Could you check a few things on this model? Use its own coordinates, in mm. A direction names the side the tool comes from. Give positions to 0.01 mm unless a question says otherwise; leave off trailing zeros. Answer in a Markdown table with one row per item. Add a question column.
1. I'm going to push flat-ended pins straight in: pin 1 Ø10.5 at (x, y) = (16, -2) entering from -Z; pin 2 Ø5.5 at (x, y) = (13, -1) entering from +Z; pin 3 Ø3 at (x, y) = (17.5, 0.5) entering from -Z; pin 4 Ø5 at (x, z) = (-27.5, -26.5) entering from -Y. Where does each tip first touch, or does it pass through?
2. I need wall thicknesses on line 1 along X through (y, z) = (-3.75, 30.5); line 2 along Z through (x, y) = (-6.5, -10); line 3 along X through (y, z) = (-6.75, 32.5). Which ranges of each line are inside material? Lowest first, please. Write a range as from..to.
3. Thinking about a two-plate mould opening in Z: for faces 1 (the flat face through (-2, 12.7, -11)), 2 (the cylindrical face through (71.111, -0.178, 9.974)), 3 (the flat face through (15, 0, -5.08)), which applies, released by +Z, released by -Z, zero draft, split by the parting line, or undercut?
4. Which directions (+Z, -Z, +X, -X, +Y, -Y) give clear straight access to the entire face, cutting with the end or side of a thin tool? Please do faces 4 (the flat face through (28.123, -0.178, -27.237)), 5 (the flat face through (-2, -12.7, -11)).
5. If we section it at A-A on z = 2.5: Count the separate pieces of the cut face and the enclosed holes in it, then the cut area to 3 significant figures.
```python
from build123d import *

# Parameters (mm, degrees)
F0_R     = 67.8507584939
F1_DEPTH = 12.7
F2_DEPTH = 12.7
F3_DEPTH = 12.7


# Not quite as in the source:
# - a feature of the source that left no trace in its solid (it failed there, or was rolled back) is left out


with BuildPart() as f1:
    # F0 (on Front) → F1 (new body, symmetric)
    with BuildSketch(Plane.XZ):
        with Locations((6.3937897791, -10.4070244153)):
            Circle(F0_R)
        with BuildLine():
            Line((16.2108500706, 8.0759122229), (29.7189755197, 33.5081515453))
            add(Edge.make_bspline(
                [(29.7189755197, 33.5081515453), (93.8960388303, -7.9348757863), (29.3413570435, -80.48370842), (-12.8972016539, -46.7268759549)],
                knots=[0, 0, 0, 0, 90.8504165915, 90.8504165915, 90.8504165915, 90.8504165915], degree=3))
            Line((-12.8972016539, -46.7268759549), (3.6481818786, -15.5762803179))
            Line((3.6481818786, -15.5762803179), (9.2231951319, -5.08))
            Line((9.2231951319, -5.08), (16.2108500706, 8.0759122229))
        make_face(mode=Mode.SUBTRACT)
        with BuildLine():
            Line((9.4068207245, 36.2007932827), (-29.3430900942, -32.6330686977))
            add(Edge.make_bspline(
                [(-29.3430900942, -32.6330686977), (-49.592975527, 0), (-23.1433883309, 42.9805777967), (9.4068207245, 36.2007932827)],
                knots=[0, 0, 0, 0, 78.9914941218, 78.9914941218, 78.9914941218, 78.9914941218], degree=3))
        make_face(mode=Mode.SUBTRACT)
    extrude(amount=F1_DEPTH, both=True)

    # F0 (on Front) → F2 (join, symmetric)
    with BuildSketch(Plane.XZ):
        Polygon((37.6452035187, -1.8549078334), (29.7189755197, 33.5081515453), (16.2108500706, 8.0759122229), (20.6487422011, -5.08), (24.1894590312, -15.5762803179), (32.1680679917, -39.2284728587), (45.5714315176, -37.2179672122), align=None)
    extrude(amount=F2_DEPTH, both=True)

    # F0 (on Front) → F3 (join, symmetric)
    with BuildSketch(Plane.XZ):
        Polygon((20.6487422011, -5.08), (9.2231951319, -5.08), (3.6481818786, -15.5762803179), (24.1894590312, -15.5762803179), align=None)
    extrude(amount=F3_DEPTH, both=True)


solid = f1.part
```
Results:
| question | item | result |
|---|---|---|
| 1 | pin 1 | z = -78.12 |
| 1 | pin 2 | z = 57.33 |
| 1 | pin 3 | z = -77.57 |
| 1 | pin 4 | y = -12.7 |
| 2 | line 1 | -47.74..-17.13, 6.2..30.39, 34.08..60.53 |
| 2 | line 2 | -77.02..-50.96, -34.68..7.94, 35.63..56.21 |
| 2 | line 3 | -46.17..-13.95, 7.32..29.94, 31.25..58.96 |
| 3 | face 1 | zero draft |
| 3 | face 2 | split by the parting line |
| 3 | face 3 | undercut |
| 4 | face 4 | +Y, -Y |
| 4 | face 5 | +Z, -Z, +X, -X, -Y |
| 5 | separate pieces | 4 |
| 5 | enclosed holes | 0 |
| 5 | area | 2,140 mm2 |
